Answer from the drawing. Dimensions are ordinates in mm from the lowest x, y and z of the part. Coordinates: 2 decimals unless noted, no trailing zeros. Order: outer loops, then holes, each group sorted by start corner. A loop starts at its lowest first (then second) coordinate and runs counter-clockwise, first axis right, second up. Notation, with made-up numbers: (25, 67.5) - (42, 67.5) arc R9 ccw to (42, 77.5) - close; hole circle Ø1 at (-24, -38.5). An arc over 180 degrees is marked (long way). One line per item, written item: value. Start each with the question number.
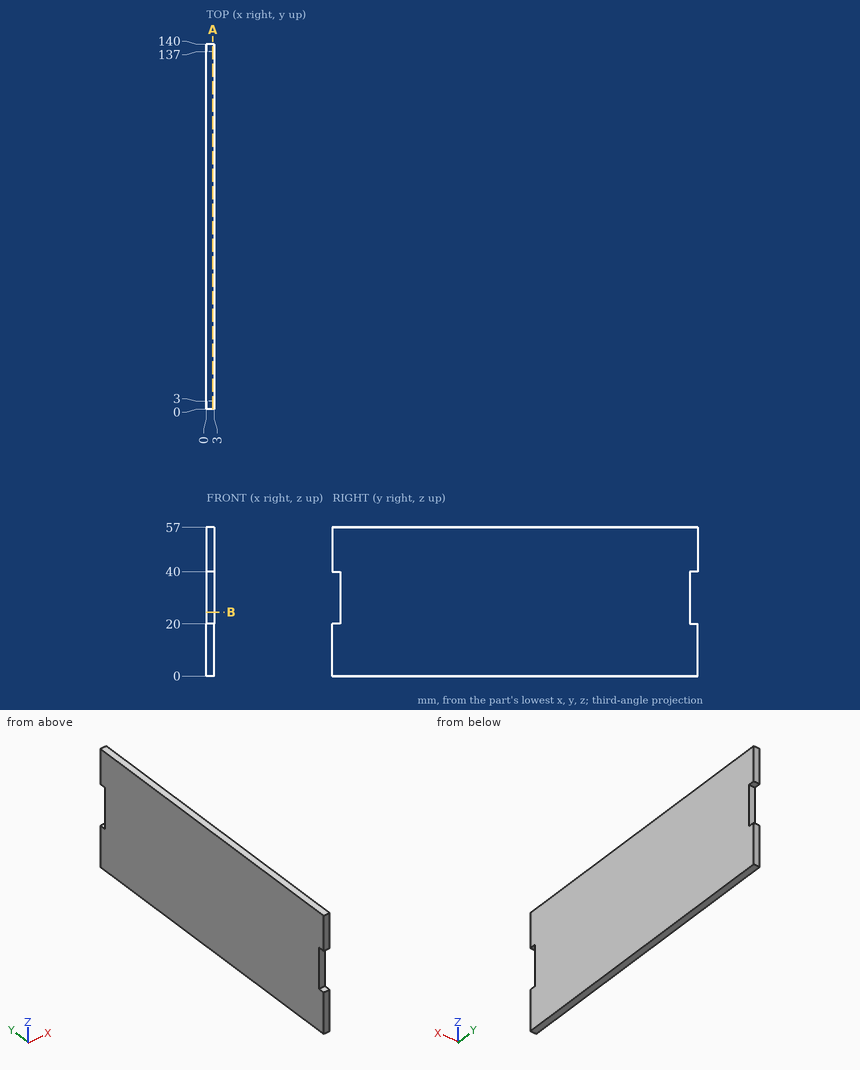
(1) Flat-ended cylindrical pins translate along their axes: pin 1 Ø1.5 at (x, y) = (2, 138.5) entering from -Z; pin 2 Ø1.5 at (x, z) = (1, 25.5) entering from +Y. Find the tip coordinate at first contact, or state that the pin passes through.
(2) The part is cut by section A-A on x = 2.5. Determine the outline of the cut face in (y, z).
(3) The part is cut by section B-B on z = 24.5. Determine the outline of the cut face in (x, y).
(4) Consider probe 1 along Y at (x, z) = (2, 25.5). Determine where the line is inside the solid, lowest interval first.
Completed:
1. pin 1: stops at z = 0
1. pin 2: stops at y = 137
2. outline: (0, 0) - (140, 0) - (140, 20) - (137, 20) - (137, 40) - (140, 40) - (140, 57) - (0, 57) - (0, 40) - (3, 40) - (3, 20) - (0, 20) - close
3. outline: (0, 3) - (3, 3) - (3, 137) - (0, 137) - close
4. probe 1: y = 3 to 137
